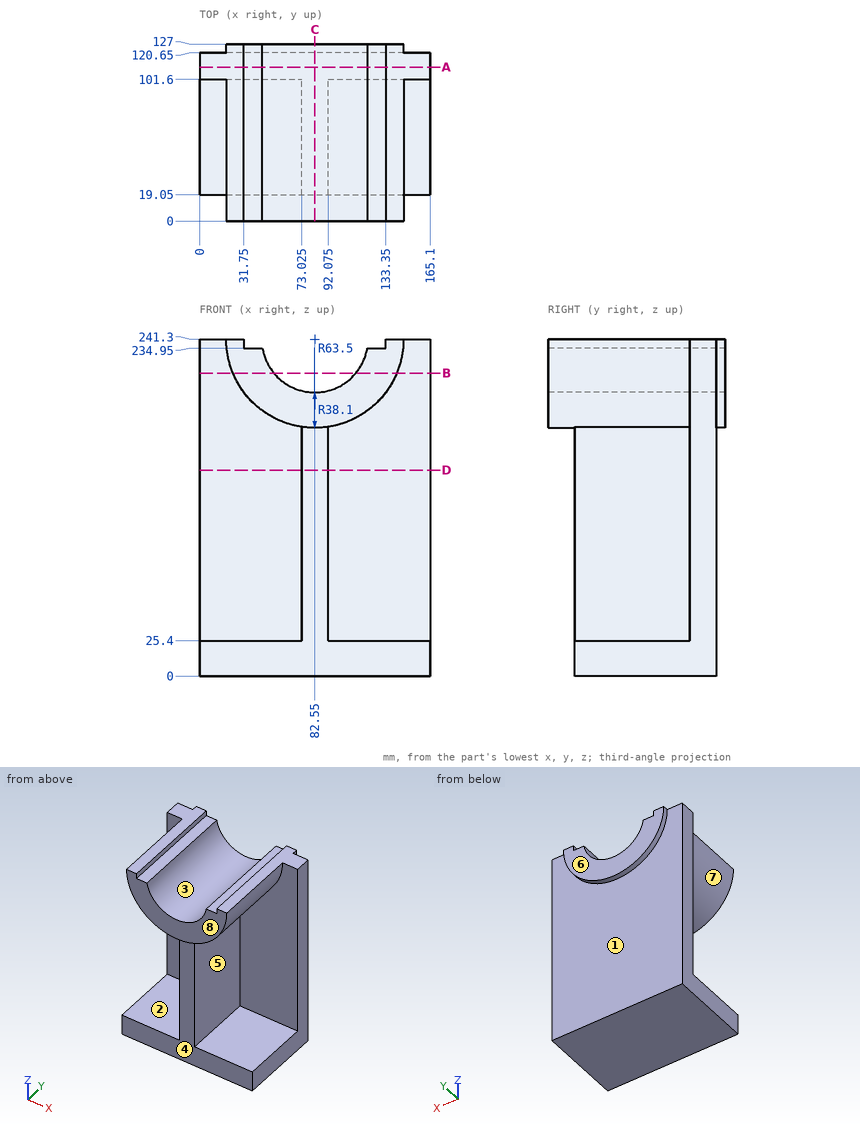
The drawing under review shows one solid part. Ordinate dimensions are in mm from its lowest x, y, z. A direction names the side the tool comes from. Give positions to 0.01 mm unless a question says otherwise; leave off trailing zeros. Write each loop counter-clockwise with the first axis right and the second up, starting at its lowest first coordinate (ties: lowest second). Pieces come first, ordered by that corner, then holes. Notation, with made-up numbers: (-12.5, 33.5) -> (26.5, 33.5) arc R18 ccw to (26.5, 43.5) -> close; hole circle Ø8 at (19.25, -5). An arc over 180 degrees is marked (long way). Use CSV: the item, a comma, the result in double quotes.
Q1. Take a section at B-B, the plane z = 217. Write out the cut boundary in (x, y).
Conclusion:
outline,"(0, 101.6) -> (23.88, 101.6) -> (23.88, 0) -> (53.21, 0) -> (53.21, 127) -> (23.88, 127) -> (23.88, 120.65) -> (0, 120.65) -> close; (111.89, 0) -> (141.22, 0) -> (141.22, 101.6) -> (165.1, 101.6) -> (165.1, 120.65) -> (141.22, 120.65) -> (141.22, 127) -> (111.89, 127) -> close"
Q2. To check wall thickness, follow probe 1 along X at (y, z) = (75, 80.5) (3 decimals); probe 2 along Y at (x, z) = (38, 128); probe 3 along Z at (x, y) = (60, 98). State the ranges of each line that lie inside material, in increasing order. Write a range as [from, to].
Conclusion:
probe 1,"[73.025, 92.075]"
probe 2,"[101.6, 120.65]"
probe 3,"[0, 25.4], [181.94, 210.59]"
Q3. For P1, Ø4, axis at x = 120.5, z = 85, coming from the -Y side; P2, Ø7, axis at y = 55, z = 237.5, coming from the +X side; P3, Ø25, axis at y = 57, z = 78.5, coming from the -X side (3 decimals); P4, Ø6, axis at x = 17, y = 103.5, coming from the -Z side, all flat-tipped, find the tip position at first contact; note any pin that passes through.
Conclusion:
P1,"y = 101.6"
P2,"x = 146.05"
P3,"x = 73.025"
P4,"z = 0"
Q4. Take a section at C-C, the plane x = 82.55. Write out the cut boundary in (y, z), then the cut area to 3 significant figures.
Conclusion:
outline,"(0, 177.8) -> (19.05, 177.8) -> (19.05, 0) -> (120.65, 0) -> (120.65, 177.8) -> (127, 177.8) -> (127, 203.2) -> (0, 203.2) -> close"
area,"21,300 mm2"
Q5. Tool access review of the marked faces 4, 5, 6, 7 and 8: name each direction out of +Z, -Z, +X, -X, +Y, -Y from which nothing blocks a thin tool from reaching the whole face with its end or side.
Conclusion:
face 4,"-Z, +X, -X, -Y"
face 5,"+X, -Y"
face 6,"+Z, -Z, +X, -X, +Y"
face 7,"-Y"
face 8,"+Z, -Z, +X, -X, -Y"
Q6. Mouldability with a two-part tool opening along Z and no side actions: class the marked faces 1, 2 and 3 as pulls with the +Z half, pulls with the -Z half, needs draft (parallel to the pull), parting line crosses it, or undercut.
Conclusion:
face 1,"needs draft"
face 2,"undercut"
face 3,"pulls with the +Z half"
Q7. Take a section at A-A, the plane y = 110.5. Write out the cut boundary in (x, z), then the cut area to 3 significant figures.
Conclusion:
outline,"(0, 0) -> (165.1, 0) -> (165.1, 241.3) -> (133.35, 241.3) -> (133.35, 234.95) -> (120.12, 234.95) arc R38.1 cw to (44.98, 234.95) -> (31.75, 234.95) -> (31.75, 241.3) -> (0, 241.3) -> close"
area,"37,400 mm2"
Q8. Take a section at D-D, the plane z = 147.5. Write out the cut boundary in (x, y) (3 decimals), then the cut area to 3 significant figures.
Conclusion:
outline,"(0, 101.6) -> (73.025, 101.6) -> (73.025, 19.05) -> (92.075, 19.05) -> (92.075, 101.6) -> (165.1, 101.6) -> (165.1, 120.65) -> (0, 120.65) -> close"
area,"4,720 mm2"
